```python
from build123d import *

# Parameters (mm, degrees)
SKETCH_1_W          = 15
SKETCH_1_H          = 15
SKETCH_1_W_2        = 13
SKETCH_1_H_2        = 13
EXTRUDE_1_DEPTH     = 270
SKETCH_2_R          = 1.5
SKETCH_2_R_2        = 2.5
SKETCH_2_R_3        = 3
CUT_EXTRUDE_1_DEPTH = 271.520331953
SKETCH_3_R          = 1.5
CUT_EXTRUDE_2_DEPTH = 271.520331953


with BuildPart() as part:
    # 草图1 → 凸台-拉伸1 (new body)
    with BuildSketch(Plane(origin=(0, 0, 0), x_dir=(1, 0, 0), z_dir=(0, 1, 0))):
        Rectangle(SKETCH_1_W, SKETCH_1_H)
        Rectangle(SKETCH_1_W_2, SKETCH_1_H_2, mode=Mode.SUBTRACT)
    extrude(amount=EXTRUDE_1_DEPTH)

    # 草图2 → 切除-拉伸1 (cut, through all)
    with BuildSketch(Plane.XY.offset(7.5)):
        with Locations((0, 155)):
            Circle(SKETCH_2_R)
        with Locations((0, 115)):
            Circle(SKETCH_2_R)
        with Locations((0, 200)):
            Circle(SKETCH_2_R)
        with Locations((0, 70)):
            Circle(SKETCH_2_R)
        with Locations((0, 220)):
            Circle(SKETCH_2_R_2)
        with Locations((0, 50)):
            Circle(SKETCH_2_R_2)
        with Locations((-2, 182.5)):
            Circle(SKETCH_2_R_3)
        with Locations((-2, 87.5)):
            Circle(SKETCH_2_R_3)
    extrude(amount=-CUT_EXTRUDE_1_DEPTH, mode=Mode.SUBTRACT)

    # 草图3 → 切除-拉伸2 (cut, through all)
    with BuildSketch(Plane(origin=(7.5, 0, 0), x_dir=(0, 0, -1), z_dir=(1, 0, 0))):
        with Locations((0, 240)):
            Circle(SKETCH_3_R)
        with Locations((0, 30)):
            Circle(SKETCH_3_R)
        with Locations((0, 10)):
            Circle(SKETCH_3_R)
        with Locations((0, 260)):
            Circle(SKETCH_3_R)
    extrude(amount=-CUT_EXTRUDE_2_DEPTH, mode=Mode.SUBTRACT)


solid = part.part
```
Part model, mm, in its own coordinate system. A direction names the side the tool comes from. Coordinates: 2 decimals unless noted, no trailing zeros. Order: outer loops, then holes, each group sorted by start corner. A loop starts at its lowest first (then second) coordinate and runs counter-clockwise, first axis right, second up. Notation, with made-up numbers: (78.5, 25.5) - (118.5, 25.5) arc R8 ccw to (118.5, 30.5) - close; hole circle Ø10 at (7, 72). An arc over 180 degrees is marked (long way). Return JSON: item names as keys, results as strings. Group by question number.
Item 1: Pin check, flat tip, straight feed: pin 1 (2.5 mm diameter, centred on x = 0, y = 200, fed in from +Z). Stop position of the tip, or through.
Item 2: Cut at B-B (y = 35). List the corners of the cut face in (x, z), plus the area to 3 significant figures.
Item 3: Cut at A-A (y = 87.5). List the corners of the cut face in (x, z).
Item 4: Pull direction Y, two halves, no side cores. Call faces 1 (the face through (-7, 270, 0)), 2 (the face through (0, 133, 6.5)), 3 (the face through (-2.65, 84.57, -6.99)): pulls with the +Y half, pulls with the -Y half, needs draft (parallel to the pull), parting line crosses it, or undercut.
Item 5: Drill centre lines: probe 1 along Y at (x, z) = (-7.2, 0); probe 2 along Z at (x, y) = (-6.25, 70.5). Where is each one in solid material? Low to high. Write a range as from..to.
Item 6: Which spindle directions (+Z, -Z, +X, -X, +Y, -Y) get a long thin tool onto all of the face, cutting with end or side? Do faces 4 (the face through (0, 133, 7.5)), 5 (the face through (0, 133, -6.5)). Say none if no direction does.
Check values:
{
 "1": {"pin 1": "passes through"},
 "2": {"outline": "(-7.5, -7.5) - (7.5, -7.5) - (7.5, 7.5) - (-7.5, 7.5) - close; hole (-6.5, -6.5) - (6.5, -6.5) - (6.5, 6.5) - (-6.5, 6.5) - close", "area": "56.0 mm2"},
 "3": {"outline": "(-7.5, -7.5) - (-5, -7.5) - (-5, -6.5) - (-6.5, -6.5) - (-6.5, 6.5) - (-5, 6.5) - (-5, 7.5) - (-7.5, 7.5) - close; (1, -7.5) - (7.5, -7.5) - (7.5, 7.5) - (1, 7.5) - (1, 6.5) - (6.5, 6.5) - (6.5, -6.5) - (1, -6.5) - close"},
 "4": {"face 1": "pulls with the +Y half", "face 2": "needs draft", "face 3": "undercut"},
 "5": {"probe 1": "y = 0..8.5, 11.5..28.5, 31.5..238.5, 241.5..258.5, 261.5..270", "probe 2": "z = -7.5..-6.5, 6.5..7.5"},
 "6": {"face 4": "+Z, +X, -X, +Y, -Y", "face 5": "+Y, -Y"}
}
